from build123d import *

# Parameters (mm, degrees)
CROQUIS1_W              = 7.5
CROQUIS1_H              = 7.5
SALIENTE_EXTRUIR1_DEPTH = 7
CROQUIS1_3_W            = 7.5
CROQUIS1_3_H            = 7.5
CROQUIS1_3_W_2          = 3.35875721
CROQUIS1_3_H_2          = 3.35875721
SALIENTE_EXTRUIR2_DEPTH = 6.5


with BuildPart() as part:
    # Croquis1 → Saliente-Extruir1 (new body)
    with BuildSketch(Plane.YZ):
        Rectangle(CROQUIS1_W, CROQUIS1_H)
    extrude(amount=-SALIENTE_EXTRUIR1_DEPTH)

    # Croquis1<3> → Saliente-Extruir2 (add)
    with BuildSketch(Plane.YZ):
        Rectangle(CROQUIS1_3_W, CROQUIS1_3_H)
        Rectangle(CROQUIS1_3_W_2, CROQUIS1_3_H_2, mode=Mode.SUBTRACT)
    extrude(amount=SALIENTE_EXTRUIR2_DEPTH)


solid = part.part
Read the model definition and answer for the solid it produces. Units are mm, in the model's axes. A direction names the side the tool comes from. Round coordinates to 2 decimals unless told otherwise and drop trailing zeros. Write each loop counter-clockwise with the first axis right and the second up, starting at its lowest first coordinate (ties: lowest second). Pieces come first, ordered by that corner, then holes.
1. The part is cut by section A-A, the plane x = 1.25. Determine the outline of the cut face in (y, z), then the cut area to 3 significant figures.
2. Which of the six approach directions +Z, -Z, +X, -X, +Y, -Y give full straight-line access (tool end or side, diameter ignored) to faces 5 (the face through (0, -3.75, 0)), 6 (the face through (3, 1.679, 0))?
3. Determine the mould class of faces 1 (the face through (0, 0, -3.75)), 2 (the face through (3, 0, 1.679)), 3 (the face through (6.5, -2, 0)), 4 (the face through (0, 0, 3.75)) for opening direction Z: pulls with the +Z half, pulls with the -Z half, needs draft (parallel to the pull), parting line crosses it, or undercut.
4. The part is cut by section B-B, the plane z = -0.25. Determine the outline of the cut face in (x, y).
5. Straight lines are drawn through the part: L1, parallel to Z at x = 1.75, y = -1.25; L2, parallel to X at y = 1.25, z = 0. For each, find the intervals that lie inside material, in ascending order.
Values:
1. outline: (-3.75, -3.75) - (3.75, -3.75) - (3.75, 3.75) - (-3.75, 3.75) - close; hole (-1.68, -1.68) - (1.68, -1.68) - (1.68, 1.68) - (-1.68, 1.68) - close
1. area: 45.0 mm2
2. face 5: +Z, -Z, +X, -X, -Y
2. face 6: +X
3. face 1: pulls with the -Z half
3. face 2: undercut
3. face 3: needs draft
3. face 4: pulls with the +Z half
4. outline: (-7, -3.75) - (6.5, -3.75) - (6.5, -1.68) - (0, -1.68) - (0, 1.68) - (6.5, 1.68) - (6.5, 3.75) - (-7, 3.75) - close
5. L1: z = -3.75 to -1.68, 1.68 to 3.75
5. L2: x = -7 to 0
